Autodesk Inventor part; units mm, degrees
ref_plane "YZ Plane" through (0, 0, 0) normal (1, 0, 0) x (0, 1, 0)
ref_plane "XZ Plane" through (0, 0, 0) normal (0, 1, 0) x (-1, 0, 0)
ref_plane "XY Plane" through (0, 0, 0) normal (0, 0, 1) x (1, 0, 0)
sketch "Skizze1" plane through (0, 0, 0) normal (0, 0, 1) x (1, 0, 0)
  line L0 (-64.7, -64.7) -> (64.7, -64.7)
  line L1 (64.7, -64.7) -> (64.7, 64.7)
  line L2 (64.7, 64.7) -> (-64.7, 64.7)
  line L3 (-64.7, 64.7) -> (-64.7, -64.7)
  line L4 (-64.7, -64.7) -> (64.7, 64.7) construction
  line L5 (64.7, -64.7) -> (-64.7, 64.7) construction
  point P0 (0, 0)
  dimension "d0" = 129.4
  dimension "d1" = 129.4
extrude "Extrusion1" add sketch "Skizze1" along normal blind 22
sketch "Skizze2" plane through (0, 0, 22) normal (0, 0, 1) x (1, 0, 0)
  line L0 (-132.05, 89.45) -> (128.95, 89.45)
  line L1 (64.7, 64.7) -> (-64.7, 64.7)
  line L2 (89.45, 116.05) -> (89.45, -84.95)
  line L3 (-89.45, 121.95) -> (-89.45, -89.05)
  line L4 (64.7, -64.7) -> (64.7, 64.7)
  line L5 (-64.7, 64.7) -> (-64.7, -64.7)
  line L6 (-157.95, -91.45) -> (148.05, -91.45)
  line L7 (-64.7, -64.7) -> (64.7, -64.7)
  line L8 (89.45, -84.95) -> (89.45, -91.95)
  line L9 (-89.45, -89.05) -> (-89.45, -94.05)
  point P0 (0, 0)
  point P1 (-89.45, -91.45)
  point P2 (89.45, -91.45)
  point P3 (89.45, 89.45)
  point P4 (-89.45, 89.45)
  dimension "d4" = 24.75
  dimension "d5" = 24.75
  dimension "d6" = 24.75
  dimension "d7" = 26.75
extrude "Extrusion2" add sketch "Skizze2" along normal blind 2 contours L0 L2 L8 L6 L9 L3 | L4 L7 L5 L1
sketch "Skizze3" plane through (0, 0, 24) normal (0, 0, 1) x (1, 0, 0)
  line L0 (-91.45, 91.45) -> (91.45, 91.45)
  line L1 (91.45, 91.45) -> (91.45, -93.45)
  line L2 (91.45, -93.45) -> (-91.45, -93.45)
  line L3 (-91.45, -93.45) -> (-91.45, 91.45)
  line L4 (89.45, 89.45) -> (-89.45, 89.45)
  line L5 (-89.45, 89.45) -> (-89.45, -91.45)
  line L6 (89.45, -91.45) -> (89.45, 89.45)
  line L7 (-89.45, -91.45) -> (89.45, -91.45)
  line L8 (-89.45, 89.45) -> (-89.45, -91.45)
  line L9 (-89.45, 89.45) -> (89.45, 89.45)
  line L10 (89.45, 89.45) -> (89.45, -91.45)
  line L11 (89.45, -91.45) -> (-89.45, -91.45)
  line L12 (-89.45, -91.45) -> (-89.45, 89.45)
  point P0 (0, 0)
  dimension "d10" = 2
  dimension "d11" = 2
  dimension "d12" = 2
  dimension "d13" = 2
extrude "Extrusion3" add sketch "Skizze3" against normal blind 10
sketch "Skizze4" plane through (0, 0, 14) normal (0, 0, -1) x (-1, 0, 0)
  line L0 (89.45, -91.45) -> (-89.45, -91.45)
  line L1 (-91.45, -93.45) -> (91.45, -93.45)
  line L2 (89.45, -91.45) -> (64.95, -91.45)
  line L3 (64.95, -91.45) -> (64.95, -93.45)
  line L4 (64.95, -93.45) -> (89.45, -93.45)
  line L5 (89.45, -93.45) -> (89.45, -91.45)
  line L6 (-89.45, -91.45) -> (-64.95, -91.45)
  line L7 (-64.95, -91.45) -> (-64.95, -93.45)
  line L8 (-64.95, -93.45) -> (-89.45, -93.45)
  line L9 (-89.45, -93.45) -> (-89.45, -91.45)
  point P0 (0, 0)
  point P1 (89.45, -93.45)
  point P2 (-89.45, -91.45)
  point P3 (-89.45, -93.45)
  point P4 (-64.95, -93.45)
  point P5 (-64.95, -91.45)
  dimension "d16" = 24.5
  dimension "d17" = 24.5
extrude "Extrusion4" cut sketch "Skizze4" against normal up to surface (8 mm away) contours L5 L1 L3 L0 | L7 L1 L9 L0
sketch "Skizze6" plane through (91.45, -93.45, 24) normal (1, 0, 0) x (0, 0, -1)
  line L0 (10, 0) -> (10, 182.9)
  line L1 (0, 0) -> (10, 0)
  line L2 (10, 0) -> (10, 27)
  line L3 (10, 27) -> (0, 27)
  line L4 (0, 27) -> (0, 0)
  line L5 (0, 184.9) -> (10, 184.9)
  line L6 (0, 184.9) -> (10, 184.9)
  line L7 (10, 184.9) -> (10, 157.9)
  line L8 (10, 157.9) -> (0, 157.9)
  line L9 (0, 157.9) -> (0, 184.9)
  point P0 (24, 93.45)
  dimension "d20" = 27
  dimension "d21" = 27
extrude "Extrusion5" cut sketch "Skizze6" against normal up to surface (2 mm away)
sketch "Skizze7" plane through (-91.45, 91.45, 24) normal (0, 1, 0) x (1, 0, 0)
  line L0 (182.9, 10) -> (180.9, 10)
  line L1 (180.9, 10) -> (180.9, 2)
  line L2 (180.9, 0) -> (0, 0)
  line L3 (182.9, 10) -> (182.9, 0)
  line L4 (181.15, 2) -> (156.65, 2)
  line L5 (156.65, 2) -> (156.65, 10)
  line L6 (156.65, 10) -> (181.15, 10)
  line L7 (181.15, 10) -> (181.15, 2)
  line L8 (180.9, 10) -> (2, 10)
  line L9 (0, 0) -> (0, 10)
  line L10 (1.75, 2) -> (26, 2)
  line L11 (26, 2) -> (26, 10)
  line L12 (26, 10) -> (1.75, 10)
  line L13 (1.75, 10) -> (1.75, 2)
  point P0 (91.45, 24)
  point P1 (181.15, 10)
  point P2 (1.75, 10)
  point P3 (2, 10)
  point P4 (180.9, 10)
  dimension "d26" = 1.75
  dimension "d27" = 24.25
  dimension "d28" = 1.75
  dimension "d29" = 2
  dimension "d30" = 1.75
  dimension "d31" = 2
  dimension "d32" = 1.75
  dimension "d33" = 24.25
extrude "Extrusion6" cut sketch "Skizze7" against normal blind 2 contours L11 L10 L13 L12 L8 | L1 L4 L5 L6
sketch "Skizze8" plane through (91.45, -66.45, 24) normal (1, 0, 0) x (0, 0, -1)
  line L0 (10, -27) -> (2, -27)
  line L1 (0, 157.9) -> (10, 157.9)
  line L2 (10, -27) -> (0, -27)
  line L3 (0, -27) -> (0, 157.9)
  line L4 (0, 157.9) -> (10, 157.9)
  line L5 (10, 157.9) -> (10, -27)
  point P0 (24, 66.45)
extrude "Extrusion7" add sketch "Skizze8" against normal blind 2
sketch "Skizze18" plane through (-91.45, -93.45, 24) normal (-1, 0, 0) x (0, 0, 1)
  line L0 (-24, 93.45) -> (0, 93.45)
  line L1 (0, 93.45) -> (0, 101.45)
  line L2 (0, 101.45) -> (-24, 101.45)
  line L3 (-24, 101.45) -> (-24, 93.45)
  dimension "d97" = 24
  dimension "d98" = 8
extrude "Extrusion17" cut sketch "Skizze18" against normal blind 35
properties part number "2025_03_10_Reaktor_oben" material "ABS-Kunststoff"
The model under review builds one solid part; all positions refer to its coordinate system, in mm. A direction names the side the tool comes from. Round coordinates to 2 decimals unless told otherwise and drop trailing zeros. Write each loop counter-clockwise with the first axis right and the second up, starting at its lowest first coordinate (ties: lowest second). Pieces come first, ordered by that corner, then holes. Notation, with made-up numbers: (-17.5, 21) - (34.5, 21) arc R27 cw to (34.5, 51) - close; hole circle Ø8 at (26.25, -1). An arc over 180 degrees is marked (long way). One line per item, written item: value. Start each with the question number.
1. Consider section A-A on x = -69. Write out the cut boundary in (y, z), and give its area (3 significant figures).
2. Consider section C-C on y = 75. Write out the cut boundary in (x, z).
3. Consider section D-D on x = 46. Write out the cut boundary in (y, z), and give its area (3 significant figures).
4. The part is to be moulded in two halves that separate along X. For faces 5 (the face through (81, 0, 22)), 6 (the face through (-89.45, -46, 18)), 7 (the face through (-91.45, -47, 19)), 8 (the face through (-1, 1, 0)), say which applies: released by +X, released by -X, zero draft, split by the parting line, or undercut.
5. To check wall thickness, follow L1, parallel to X at y = 54.5, z = 19.75; L2, parallel to Y at x = -13, z = 15.25; L3, parallel to X at y = 71.5, z = 21.75. State the ranges of each line that lie inside material, in increasing order. Write a range as from..to.
6. Consider section B-B on z = 19.75. State how many separate pieces and enclosed holes the cut face has, and give its area (3 significant figures).
7. Clearance check with flat-ended pins moving along their axes: P1, Ø4, axis at y = -67, z = 11, coming from the -X side; P2, Ø8, axis at y = -7.5, z = 8.5, coming from the +X side; P3, Ø2, axis at x = -3, y = 91, coming from the -Z side; P4, Ø1, axis at x = -9, z = 10, coming from the -Y side. State where each tip first meets the part, or that it passes through.
8. Machinability: for faces 1 (the face through (-64, 0, 15)), 2 (the face through (-1, 91.45, 19)), 3 (the face through (-64.7, -32, 11)), 4 (the face through (89.45, 0, 18)), which of the approach directions +Z, -Z, +X, -X, +Y, -Y give a long, thin tool a straight path to every point of the face, cutting with its end or side? Answer none if there is none.
Checks:
1. outline: (-93.45, 22) - (0, 22) - (0, 24) - (-93.45, 24) - close; (8, 22) - (91.45, 22) - (91.45, 24) - (8, 24) - close
1. area: 354 mm^2
2. outline: (-91.45, 14) - (-89.45, 14) - (-89.45, 22) - (89.45, 22) - (89.45, 14) - (91.45, 14) - (91.45, 24) - (-91.45, 24) - close
3. outline: (-93.45, 14) - (-91.45, 14) - (-91.45, 22) - (-64.7, 22) - (-64.7, 0) - (64.7, 0) - (64.7, 22) - (89.45, 22) - (89.45, 14) - (91.45, 14) - (91.45, 24) - (-93.45, 24) - close
3. area: 3,250 mm^2
4. face 5: undercut
4. face 6: undercut
4. face 7: released by -X
4. face 8: zero draft
5. L1: x = -91.45..-89.45, -64.7..64.7, 89.45..91.45
5. L2: y = -93.45..-91.45, -64.7..64.7, 89.45..91.45
5. L3: x = -91.45..-89.45, 89.45..91.45
6. separate pieces: 6
6. enclosed holes: 0
6. area: 17,900 mm^2
7. P1: passes through
7. P2: stops at x = 64.7
7. P3: stops at z = 14
7. P4: stops at y = -64.7
8. face 1: +Z, -Z, -X
8. face 2: +Z, -Z, +X, -X, +Y
8. face 3: -Z
8. face 4: -Z, +Y, -Y
